Model file for the job. Use its own axes, mm. Face numbers are marked on the shaded views. Round coordinates to 2 decimals unless told otherwise and drop trailing zeros. Order: outer loops, then holes, each group sorted by start corner. A loop starts at its lowest first (then second) coordinate and runs counter-clockwise, first axis right, second up. Notation, with made-up numbers: (-35.75, 32) -> (-24.75, 32) arc R18 ccw to (-24.75, 66) -> close; hole circle Ø1 at (-27, 3.25). An arc over 180 degrees is marked (long way). Put each result on its own line as item: value. Start each with the question number.
Q1. Probe L1, parallel to Y at x = -1.75, z = 7.25; L2, parallel to X at y = 82, z = -4.25; L3, parallel to Y at x = 0, z = -2.5 (3 decimals). List the from-to ranges inside material, lowest first.
Q2. Flat gauge pins, fed straight in: P1, Ø4.5, axis at y = 32.5, z = 2.5, coming from the +X side; P2, Ø1.5, axis at x = -2, z = 0.5, coming from the -Y side; P3, Ø4.5, axis at x = 0, y = 0, coming from the -Z side. Where does each tip first touch, or does it go through?
Q3. Pull direction Y, two halves, no side cores. Call the marked faces 1 and 2: released by +Y, released by -Y, zero draft, split by the parting line, or undercut.
Q4. Cut at C-C, the plane x = 1. State how many separate pieces and enclosed holes the cut face has, and give its area (3 significant figures).
Q5. Cut at B-B, the plane y = 71.5. List the corners of the cut face in (x, z), and give its area (3 significant figures).
Q6. Cut at A-A, the plane z = -2. List the corners of the cut face in (x, y) (3 decimals).
from build123d import *

# Parameters (mm, degrees)
SKETCH1_R             = 2.025
BOSS_EXTRUDE1_DEPTH   = 9
BOSS_EXTRUDE2_START   = -15
SKETCH2_R             = 5
SKETCH2_R_2           = 2.025
BOSS_EXTRUDE2_DEPTH   = 15
BOSS_EXTRUDE3_START   = -12
SKETCH3_R             = 2.025
BOSS_EXTRUDE3_DEPTH   = 12
CROQUIS1_W            = 6
CROQUIS1_H            = 12.01125174
CORTAR_EXTRUIR3_DEPTH = 10
REDONDEO1_R           = 1
REDONDEO2_R           = 1


with BuildPart() as part:
    # Sketch1 → Boss-Extrude1 (new body)
    with BuildSketch(Plane.XY):
        with BuildLine():
            Line((-5, 0), (-5, 85))
            ThreePointArc((-5, 85), (3.535533906, 88.535533906), (0, 80))
            Line((0, 80), (0, 5))
            ThreePointArc((0, 5), (5, 0), (0, -5))
            ThreePointArc((0, -5), (-3.535533906, -3.535533906), (-5, 0))
        make_face()
        with Locations((0, 85)):
            Circle(SKETCH1_R, mode=Mode.SUBTRACT)
        Circle(SKETCH1_R, mode=Mode.SUBTRACT)
    extrude(amount=BOSS_EXTRUDE1_DEPTH)

    # Sketch2 → Boss-Extrude2 (add)
    with BuildSketch(Plane.XY.offset(9).offset(BOSS_EXTRUDE2_START)):
        with Locations(Location((0, 85, 0), (0, 0, 180))):
            Circle(SKETCH2_R)
        with Locations((0, 85)):
            Circle(SKETCH2_R_2, mode=Mode.SUBTRACT)
    extrude(amount=BOSS_EXTRUDE2_DEPTH)

    # Sketch3 → Boss-Extrude3 (add)
    with BuildSketch(Plane.XY.offset(9).offset(BOSS_EXTRUDE3_START)):
        with BuildLine():
            Line((-5, 0), (-5, 85))
            ThreePointArc((-5, 85), (-4.183300133, 82.261387212), (-2, 80.417424305))
            Line((-2, 80.417424305), (-2, 5))
            Line((-2, 5), (0, 5))
            ThreePointArc((0, 5), (5, 0), (0, -5))
            ThreePointArc((0, -5), (-3.535533906, -3.535533906), (-5, 0))
        make_face()
        Circle(SKETCH3_R, mode=Mode.SUBTRACT)
    extrude(amount=BOSS_EXTRUDE3_DEPTH)

    # Croquis1 → Cortar-Extruir3 (cut)
    with BuildSketch(Plane.ZY.offset(5)):
        with Locations((0, 1.00562587)):
            Rectangle(CROQUIS1_W, CROQUIS1_H)
    extrude(amount=-CORTAR_EXTRUIR3_DEPTH, mode=Mode.SUBTRACT)

    # Redondeo1
    redondeo1_edges = [part.edges().sort_by_distance(p)[0] for p in [
        (-1.021548218, 80.105468435, 0),
        (-2, 43.714338023, 0),
    ]]
    fillet(redondeo1_edges, radius=REDONDEO1_R)

    # Redondeo2
    redondeo2_edges = [part.edges().sort_by_distance(p)[0] for p in [
        (0, 42.5, 9),
        (3.535533906, 88.535533906, 9),
        (-5, 42.5, 9),
        (3.535533906, -3.535533906, 9),
    ]]
    fillet(redondeo2_edges, radius=REDONDEO2_R)


solid = part.part
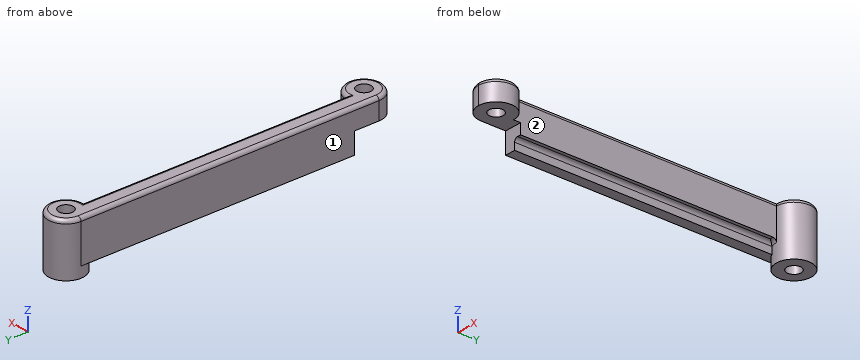
Ans:
1. L1: y = -4.68 to -1.02, 1.02 to 83.98, 86.02 to 89.68
1. L2: x = -4 to 4
1. L3: y = 80 to 82.975, 87.025 to 90
2. P1: stops at x = 0
2. P2: stops at y = 7.01
2. P3: stops at z = 3
3. face 1: zero draft
3. face 2: undercut
4. separate pieces: 4
4. enclosed holes: 0
4. area: 131 mm^2
5. outline: (-5, -3) -> (-2, -3) -> (-2, -1) arc R1 cw to (-1, 0) -> (0, 0) -> (0, 8) arc R1 ccw to (-1, 9) -> (-4, 9) arc R1 ccw to (-5, 8) -> close
5. area: 53.8 mm^2
6. outline: (-5, 7.011) -> (-2, 7.011) -> (-2, 80.417) arc R5 ccw (long way) to (-5, 85) -> close; hole circle Ø4.05 at (0, 85)
